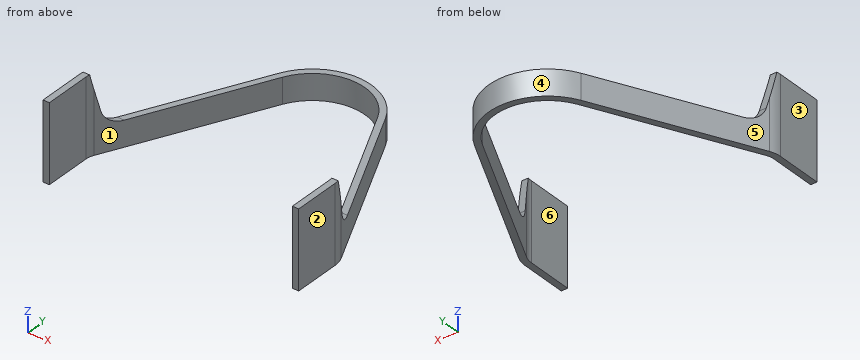
from build123d import *

# Parameters (mm, degrees)
EXTRUDE_1_DEPTH     = 121
CUT_EXTRUDE_1_DEPTH = 506.269235161


with BuildPart() as part:
    # 草图1 → 凸台-拉伸1 (new body)
    with BuildSketch(Plane.XY):
        with BuildLine():
            Line((-190, -210.857487736), (-190, -284))
            Line((-190, -284), (-200, -284))
            Line((-200, -284), (-200, -210.857487736))
            ThreePointArc((-200, -210.857487736), (-198.994242885, -201.944069658), (-196.027548908, -193.478888262))
            Line((-196.027548908, -193.478888262), (-83.313706851, 40.188011282))
            ThreePointArc((-83.313706851, 40.188011282), (0, 92.5), (83.313706851, 40.188011282))
            Line((83.313706851, 40.188011282), (196.027548908, -193.478888262))
            ThreePointArc((196.027548908, -193.478888262), (198.994242885, -201.944069658), (200, -210.857487736))
            Line((200, -210.857487736), (200, -284))
            Line((200, -284), (190, -284))
            Line((190, -284), (190, -210.857487736))
            ThreePointArc((190, -210.857487736), (189.245682164, -204.172424177), (187.020661681, -197.82353813))
            Line((187.020661681, -197.82353813), (74.306819623, 35.843361414))
            ThreePointArc((74.306819623, 35.843361414), (0, 82.5), (-74.306819623, 35.843361414))
            Line((-74.306819623, 35.843361414), (-187.020661681, -197.82353813))
            ThreePointArc((-187.020661681, -197.82353813), (-189.245682164, -204.172424177), (-190, -210.857487736))
        make_face()
    extrude(amount=EXTRUDE_1_DEPTH)

    # 草图2 → 切除-拉伸1 (cut, through all)
    with BuildSketch(Plane.ZY.offset(200)):
        with BuildLine():
            Line((40, 92.5), (40, -160.506441654))
            ThreePointArc((40, -160.506441654), (46.380696587, -179.003157748), (62.808567085, -189.631744959))
            Line((62.808567085, -189.631744959), (121, -204))
            Line((121, -204), (121, 92.5))
            Line((121, 92.5), (40, 92.5))
        make_face()
    extrude(amount=-CUT_EXTRUDE_1_DEPTH, mode=Mode.SUBTRACT)


solid = part.part
Read the model definition and answer for the solid it produces. Units are mm, in the model's axes. Face numbers are marked on the shaded views. A direction names the side the tool comes from. Give positions to 0.01 mm unless a question says otherwise; leave off trailing zeros. Write each loop counter-clockwise with the first axis right and the second up, starting at its lowest first coordinate (ties: lowest second). Pieces come first, ordered by that corner, then holes. Notation, with made-up numbers: (15.5, 9.25) - (59.5, 9.25) arc R25 cw to (59.5, 35.25) - close; hole circle Ø4 at (77, -18.75). An arc over 180 degrees is marked (long way). Use CSV: the item, a comma, the result in double quotes. Start each with the question number.
(1) For the marked faces 5 and 6, determine the directions among +Z, -Z, +X, -X, +Y, -Y from which every point of the face is accessible in a straight line to the end or side of a thin tool.
(2) Find section C-C (z = 23). Give the vertices of the cut face in (x, y), plus the area to 3 significant figures.
(3) Determine the mould class of the marked faces 1, 2, 3 and 4 for opening direction X: +X half, -X half, draft (parallel to the pull), parting line (faces both ways), or undercut.
(4) Find section B-B (z = 110). Give the vertices of the cut face in (x, y), plus the area to 3 significant figures.
(5) Consider line 1 along X through (y, z) = (5, 15); line 2 along Y through (x, z) = (-72.5, 31); line 3 along Z through (x, y) = (88, 11). Determine where each line is inside the solid, lowest interval first.
(6) Given P1, Ø1, axis at y = -130.5, z = 39.5, coming from the +X side; P2, Ø1.5, axis at x = -113, z = 33, coming from the +Y side, each flat-ended and moving along its own axis, determine where each tip first touches the part or whether it passes through.
(7) Find section D-D (z = 49.5). Give the vertices of the cut face in (x, y).
(8) Find section A-A (y = -256). Give the vertices of the cut face in (x, z), plus the area to 3 significant figures.
Findings below:
1,face 5,"+Z, -Z, -X, +Y"
1,face 6,"+Z, -Z, -Y"
2,outline,"(-200, -284) - (-190, -284) - (-190, -210.86) arc R30 cw to (-187.02, -197.82) - (-74.31, 35.84) arc R82.5 cw to (74.31, 35.84) - (187.02, -197.82) arc R30 cw to (190, -210.86) - (190, -284) - (200, -284) - (200, -210.86) arc R40 ccw to (196.03, -193.48) - (83.31, 40.19) arc R92.5 ccw to (-83.31, 40.19) - (-196.03, -193.48) arc R40 ccw to (-200, -210.86) - close"
2,area,"8,930 mm2"
3,face 1,"undercut"
3,face 2,"+X half"
3,face 3,"-X half"
3,face 4,"parting line"
4,outline,"(-200, -284) - (-190, -284) - (-190, -210.86) arc R30 cw to (-188.43, -201.28) - (-198.84, -201.28) arc R40 ccw to (-200, -210.86) - close; (188.43, -201.28) arc R30 cw to (190, -210.86) - (190, -284) - (200, -284) - (200, -210.86) arc R40 ccw to (198.84, -201.28) - close"
4,area,"1,660 mm2"
5,line 1,"-100.29 to -89.18, 89.18 to 100.29"
5,line 2,"39.37 to 57.45"
5,line 3,"0 to 40"
6,P1,"x = 165.89"
6,P2,"y = -19.8"
7,outline,"(-200, -284) - (-190, -284) - (-190, -210.86) arc R30 cw to (-187.02, -197.82) - (-179.59, -182.41) - (-190.69, -182.41) - (-196.03, -193.48) arc R40 ccw to (-200, -210.86) - close; (179.59, -182.41) - (187.02, -197.82) arc R30 cw to (190, -210.86) - (190, -284) - (200, -284) - (200, -210.86) arc R40 ccw to (196.03, -193.48) - (190.69, -182.41) - close"
8,outline,"(-200, 0) - (-190, 0) - (-190, 121) - (-200, 121) - close; (190, 0) - (200, 0) - (200, 121) - (190, 121) - close"
8,area,"2,420 mm2"
